Model file for the job. Use its own axes, mm. Round coordinates to 2 decimals unless told otherwise and drop trailing zeros. Order: outer loops, then holes, each group sorted by start corner. A loop starts at its lowest first (then second) coordinate and runs counter-clockwise, first axis right, second up. Notation, with made-up numbers: (0.5, -30) - (12.5, -30) arc R36 cw to (12.5, 7) - close; hole circle Ø9 at (-13, -20). An arc over 180 degrees is marked (long way). Write item = value, one per line.
```python
from build123d import *

# Parameters (mm, degrees)
SKETCH1_R           = 4
SKETCH1_R_2         = 3.15
SKETCH1_R_3         = 1.65
SKETCH1_R_4         = 1.5
SKETCH1_R_5         = 11
BOSS_EXTRUDE1_DEPTH = 2


with BuildPart() as part:
    # Sketch1 → Boss-Extrude1 (new body)
    with BuildSketch(Plane.XY):
        with BuildLine():
            ThreePointArc((-137, 0), (-133.485281374, -8.485281374), (-125, -12))
            Line((-125, -12), (125, -12))
            ThreePointArc((125, -12), (133.485281374, -8.485281374), (137, 0))
            Line((137, 0), (137, 180))
            Line((137, 180), (-53.998245329, 180))
            Line((-53.998245329, 180), (-137, 180))
            Line((-137, 180), (-137, 0))
        make_face()
        with Locations((-125, 0)):
            Circle(SKETCH1_R, mode=Mode.SUBTRACT)
        with Locations((-42, 0)):
            Circle(SKETCH1_R, mode=Mode.SUBTRACT)
        with Locations((42, 0)):
            Circle(SKETCH1_R, mode=Mode.SUBTRACT)
        with Locations((125, 0)):
            Circle(SKETCH1_R, mode=Mode.SUBTRACT)
        with Locations((-117, 103)):
            Circle(SKETCH1_R_2, mode=Mode.SUBTRACT)
        with Locations((-117, 120)):
            Circle(SKETCH1_R_3, mode=Mode.SUBTRACT)
        with Locations((-97, 120)):
            Circle(SKETCH1_R_3, mode=Mode.SUBTRACT)
        with Locations((-77, 120)):
            Circle(SKETCH1_R_3, mode=Mode.SUBTRACT)
        with Locations((-47, 103)):
            Circle(SKETCH1_R_2, mode=Mode.SUBTRACT)
        with Locations((-117, 140)):
            Circle(SKETCH1_R_3, mode=Mode.SUBTRACT)
        with Locations((-97, 140)):
            Circle(SKETCH1_R_3, mode=Mode.SUBTRACT)
        with Locations((-77, 140)):
            Circle(SKETCH1_R_3, mode=Mode.SUBTRACT)
        with Locations((-117, 160)):
            Circle(SKETCH1_R_3, mode=Mode.SUBTRACT)
        with Locations((-107, 170)):
            Circle(SKETCH1_R_2, mode=Mode.SUBTRACT)
        with Locations((-97, 160)):
            Circle(SKETCH1_R_3, mode=Mode.SUBTRACT)
        with Locations((-77, 160)):
            Circle(SKETCH1_R_3, mode=Mode.SUBTRACT)
        with Locations((-5, 150)):
            Circle(SKETCH1_R, mode=Mode.SUBTRACT)
        with Locations((7, 103)):
            Circle(SKETCH1_R_2, mode=Mode.SUBTRACT)
        with Locations((31, 130)):
            Circle(SKETCH1_R_4, mode=Mode.SUBTRACT)
        with Locations((45, 116)):
            Circle(SKETCH1_R_4, mode=Mode.SUBTRACT)
        with Locations((45, 130)):
            Circle(SKETCH1_R_5, mode=Mode.SUBTRACT)
        with Locations((59, 130)):
            Circle(SKETCH1_R_4, mode=Mode.SUBTRACT)
        with Locations((117, 103)):
            Circle(SKETCH1_R_2, mode=Mode.SUBTRACT)
        with Locations((45, 144)):
            Circle(SKETCH1_R_4, mode=Mode.SUBTRACT)
        with BuildLine():
            ThreePointArc((129, 120), (125, 116), (121, 120))
            Line((121, 120), (121, 170))
            ThreePointArc((121, 170), (125, 174), (129, 170))
            Line((129, 170), (129, 120))
        make_face(mode=Mode.SUBTRACT)
        with Locations((107, 170)):
            Circle(SKETCH1_R_2, mode=Mode.SUBTRACT)
    extrude(amount=BOSS_EXTRUDE1_DEPTH)


solid = part.part
```
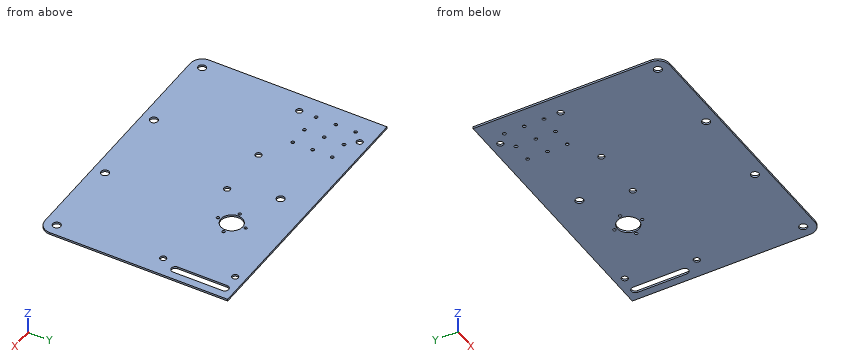
1) Cut at B-B (x = 117). Write the cut outline in (y, z).
Conclusion:
outline = (-12, 0) - (99.85, 0) - (99.85, 2) - (-12, 2) - close; (106.15, 0) - (180, 0) - (180, 2) - (106.15, 2) - close
2) Cut at C-C (y = 150). Write the cut outline in (x, z).
Conclusion:
outline = (-137, 0) - (-9, 0) - (-9, 2) - (-137, 2) - close; (-1, 0) - (121, 0) - (121, 2) - (-1, 2) - close; (129, 0) - (137, 0) - (137, 2) - (129, 2) - close
3) Cut at D-D (z = 1.7). Give the number of separate pieces and of enclosed holes in the cut face, and give its area (3 significant figures).
Conclusion:
separate_pieces = 1
enclosed_holes = 26
area = 51,200 mm^2
4) Cut at A-A (y = 103). Write the cut outline in (x, z), and give its area (3 significant figures).
Conclusion:
outline = (-137, 0) - (-120.15, 0) - (-120.15, 2) - (-137, 2) - close; (-113.85, 0) - (-50.15, 0) - (-50.15, 2) - (-113.85, 2) - close; (-43.85, 0) - (3.85, 0) - (3.85, 2) - (-43.85, 2) - close; (10.15, 0) - (113.85, 0) - (113.85, 2) - (10.15, 2) - close; (120.15, 0) - (137, 0) - (137, 2) - (120.15, 2) - close
area = 498 mm^2
5) Wall check: line 1 along Y through (x, z) = (125, 1.4); line 2 along Y through (x, z) = (-117, 0.8); line 3 along Y through (x, z) = (7, 1.4). Give the ranges that are in metal, low to high.
Conclusion:
line_1 = -12 to -4, 4 to 116, 174 to 180
line_2 = -12 to 99.85, 106.15 to 118.35, 121.65 to 138.35, 141.65 to 158.35, 161.65 to 180
line_3 = -12 to 99.85, 106.15 to 180
